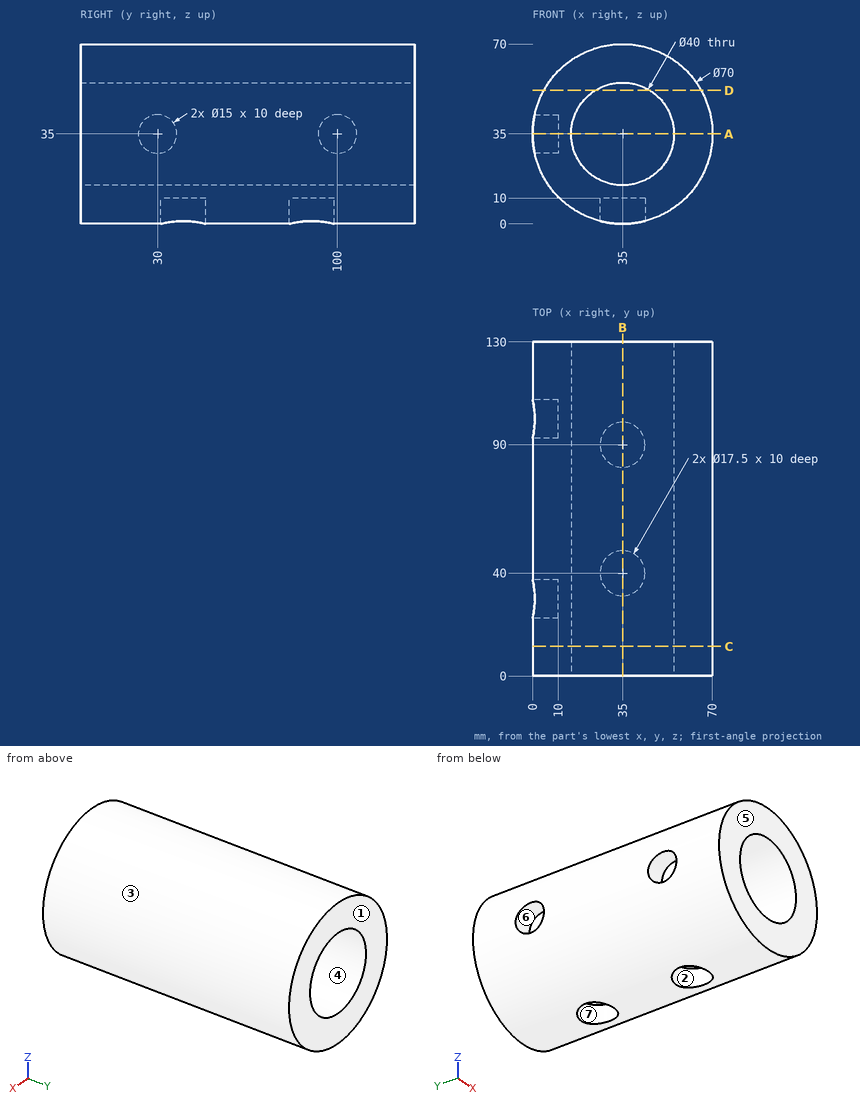
Study the drawing (mm; zero at the part's minimum x, y, z) and answer. A direction names the side the tool comes from. Round coordinates to 2 decimals unless told otherwise and drop trailing zeros. Loops run counter-clockwise (first coordinate to the right, second up) from the corner with the lowest first, then second, coordinate; pieces in that order, holes last. Notation, with made-up numbers: (7.5, -35.5) -> (35.5, -35.5) arc R27 cw to (35.5, -0.5) -> close; hole circle Ø4 at (16.25, 79.5). An arc over 180 degrees is marked (long way). One line per item, written item: value.
1) Consider L1, parallel to Y at x = 3.25, z = 35; L2, parallel to Y at x = 43, z = 9; L3, parallel to Z at x = 17, y = 119. Determine where each line is inside the solid, lowest interval first. Write a range as [from, to].
Answer list:
L1: y = [0, 22.5], [37.5, 92.5], [107.5, 130]
L2: y = [0, 36.46], [43.54, 86.46], [93.54, 130]
L3: z = [4.98, 26.28], [43.72, 65.02]
2) A cutting plane is placed at C-C (y = 11.5). Determine the outline of the cut face in (x, z).
Answer list:
outline: circle Ø70 at (35, 35); hole circle Ø40 at (35, 35)
3) A cutting plane is placed at B-B (x = 35). Determine the outline of the cut face in (y, z), and give its area (3 significant figures).
Answer list:
outline: (0, 0) -> (31.25, 0) -> (31.25, 10) -> (48.75, 10) -> (48.75, 0) -> (81.25, 0) -> (81.25, 10) -> (98.75, 10) -> (98.75, 0) -> (130, 0) -> (130, 15) -> (0, 15) -> close; (0, 55) -> (130, 55) -> (130, 70) -> (0, 70) -> close
area: 3,550 mm²
4) Flat-ended cylindrical pins translate along their axes: P1, Ø9, axis at y = 30, z = 35, coming from the +X side; P2, Ø1, axis at x = 60, y = 89, coming from the +Z side (3 decimals); P3, Ø5, axis at y = 108.5, z = 24, coming from the +X side. Find the tip coordinate at first contact, or state that the pin passes through.
Answer list:
P1: stops at x = 70
P2: stops at z = 59.995
P3: stops at x = 68.95
5) For the marked faces 5, 6 and 7, determine the directions among +Z, -Z, +X, -X, +Y, -Y from which every point of the face is accessible in a straight line to the end or side of a thin tool.
Answer list:
face 5: +Z, -Z, +X, -X, -Y
face 6: -X
face 7: -Z
6) A cutting plane is placed at A-A (z = 35). Determine the outline of the cut face in (x, y), and give its area (3 significant figures).
Answer list:
outline: (0, 0) -> (15, 0) -> (15, 130) -> (0, 130) -> (0, 107.5) -> (10, 107.5) -> (10, 92.5) -> (0, 92.5) -> (0, 37.5) -> (10, 37.5) -> (10, 22.5) -> (0, 22.5) -> close; (55, 0) -> (70, 0) -> (70, 130) -> (55, 130) -> close
area: 3,600 mm²
7) A cutting plane is placed at D-D (z = 52). Determine the outline of the cut face in (x, y).
Answer list:
outline: (4.41, 0) -> (24.46, 0) -> (24.46, 130) -> (4.41, 130) -> close; (45.54, 0) -> (65.59, 0) -> (65.59, 130) -> (45.54, 130) -> close
8) The mould has two halves that part along X. Classify the marked faces 1, 2, 3 and 4: pulls with the +X half, pulls with the -X half, needs draft (parallel to the pull), parting line crosses it, or undercut.
Answer list:
face 1: needs draft
face 2: undercut
face 3: parting line crosses it
face 4: undercut
